from build123d import *

# Parameters (mm, degrees)
BOSS_EXTRUDE1_DEPTH     = 46
CUT_EXTRUDE1_DEPTH      = 11
SKETCH3_R               = 12.5
CUT_EXTRUDE2_DEPTH      = 300.311710429
SKETCH4_R               = 12.5
BOSS_EXTRUDE2_DEPTH     = 5
CUT_EXTRUDE3_DEPTH      = 301.796442798
CUT_EXTRUDE3_DEPTH_BACK = 301.796442798
SKETCH5_R               = 12.75


with BuildPart() as part:
    # Sketch1 → Boss-Extrude1 (new body)
    with BuildSketch(Plane(origin=(0, 0, 0), x_dir=(1, 0, 0), z_dir=(0, 1, 0))):
        with BuildLine():
            Line((0, 92.5), (190, 92.5))
            ThreePointArc((190, 92.5), (282.5, 0), (190, -92.5))
            Line((190, -92.5), (0, -92.5))
            ThreePointArc((0, -92.5), (-92.5, 0), (0, 92.5))
        make_face()
    extrude(amount=BOSS_EXTRUDE1_DEPTH)

    # Sketch2 → Cut-Extrude1 (cut)
    with BuildSketch(Plane.XZ):
        with BuildLine():
            Line((80, -92.5), (80, -22.5))
            ThreePointArc((80, -22.5), (57.5, 0), (80, 22.5))
            Line((80, 22.5), (80, 92.5))
            Line((80, 92.5), (102.5, 92.5))
            Line((102.5, 92.5), (102.5, 22.5))
            ThreePointArc((102.5, 22.5), (125, 0), (102.5, -22.5))
            Line((102.5, -22.5), (102.5, -92.5))
            Line((102.5, -92.5), (80, -92.5))
        make_face()
    extrude(amount=-CUT_EXTRUDE1_DEPTH, mode=Mode.SUBTRACT)

    # Sketch3 → Cut-Extrude2 (cut, through all)
    with BuildSketch(Plane.XZ.offset(-11)):
        with Locations(Location((91.25, 0, 0), (0, 0, 270))):
            Circle(SKETCH3_R)
    extrude(amount=-CUT_EXTRUDE2_DEPTH, mode=Mode.SUBTRACT)

    # Sketch4 → Boss-Extrude2 (add)
    with BuildSketch(Plane(origin=(0, 46, 0), x_dir=(1, 0, 0), z_dir=(0, 1, 0))):
        with BuildLine():
            ThreePointArc((102.089515, 21.8501808), (124.589515, -0.6498192), (102.089515, -23.1498192))
            Line((102.089515, -23.1498192), (79.589515, -23.1498192))
            ThreePointArc((79.589515, -23.1498192), (57.089515, -0.6498192), (79.589515, 21.8501808))
            Line((79.589515, 21.8501808), (102.089515, 21.8501808))
        make_face()
        with Locations(Location((91.25, 0, 0), (0, 0, 90))):
            Circle(SKETCH4_R, mode=Mode.SUBTRACT)
    extrude(amount=BOSS_EXTRUDE2_DEPTH)

    # Sketch5 → Cut-Extrude3 (cut, two sides: drawn at the far end of the back side and taken through both)
    with BuildSketch(Plane(origin=(0, 46, 0), x_dir=(1, 0, 0), z_dir=(0, 1, 0)).offset(-CUT_EXTRUDE3_DEPTH_BACK)):
        with Locations(Location((1.25, 0, 0), (0, 0, 270))):
            Circle(SKETCH5_R)
        with Locations(Location((181.25, 0, 0), (0, 0, 270))):
            Circle(SKETCH5_R)
    extrude(amount=CUT_EXTRUDE3_DEPTH + CUT_EXTRUDE3_DEPTH_BACK, mode=Mode.SUBTRACT)


solid = part.part
Geometry check sheet. Reference: the model listing, model coordinates, mm. A direction names the side the tool comes from. Coordinates: 2 decimals unless noted, no trailing zeros. Order: outer loops, then holes, each group sorted by start corner. A loop starts at its lowest first (then second) coordinate and runs counter-clockwise, first axis right, second up. Notation, with made-up numbers: (78, 51.5) - (114, 51.5) arc R17 cw to (114, 71.5) - close; hole circle Ø11 at (-16.75, 82). An arc over 180 degrees is marked (long way). Answer in a Markdown table with one row per item. Add a question column.
1) Cross-section at B-B, the plane x = 181.25. Record the cut outline in (y, z), then the cut area to 3 significant figures.
2) Gauge pin test, flat ends, axial feed: P1, Ø5, axis at y = 31.5, z = 70.5, coming from the +X side; P2, Ø5, axis at x = 244, y = 18.5, coming from the +Z side; P3, Ø1, axis at y = 41, z = -34, coming from the -X side. Record the tip position at first contact, or that the pin passes through.
3) Material ranges on line 1 along X through (y, z) = (42, 0); line 2 along Z through (x, y) = (91, 29); line 3 along Z through (x, y) = (1.25, 30), recorded low to high. Write a range as [from, to].
4) Release check for a two-part mould opening along X. For faces 1 (the flat face through (96, 23, 92.5)), 2 (the cylindrical face through (282.478, 22.678, -2.034)), 3 (the cylindrical face through (57.095, 48.465, 1.145)), 4 (the cylindrical face through (57.505, 5.423, -0.495)) record: +X half, -X half, draft (parallel to the pull), parting line (faces both ways), or undercut.
5) Cross-section at A-A, the plane y = 6. Record the cut outline in (x, z), then the cut area to 3 significant figures.
6) Set-up check for faces 5 (the flat face through (77, 11, 1)), 6 (the cylindrical face through (124.584, 48.465, 0.155)), 7 (the flat face through (102.5, 5, -57)): record each of +Z, -Z, +X, -X, +Y, -Y from which the full face is reachable in a straight line by a thin tool's end or side.
7) Cross-section at C-C, the plane y = 22. Record the cut outline in (x, z).
8) Cross-section at D-D, the plane z = 0. Record the cut outline in (x, y).
Check result:
| question | item | result |
|---|---|---|
| 1 | outline | (0, -92.5) - (46, -92.5) - (46, -12.75) - (0, -12.75) - close; (0, 12.75) - (46, 12.75) - (46, 92.5) - (0, 92.5) - close |
| 1 | area | 7,340 mm² |
| 2 | P1 | stops at x = 252.71 |
| 2 | P2 | stops at z = 76.84 |
| 2 | P3 | stops at x = -86.22 |
| 3 | line 1 | x = [-92.5, -11.5], [14, 78.75], [103.75, 168.5], [194, 282.5] |
| 3 | line 2 | z = [-92.5, -12.5], [12.5, 92.5] |
| 3 | line 3 | z = [-92.5, -12.75], [12.75, 92.5] |
| 4 | face 1 | draft |
| 4 | face 2 | +X half |
| 4 | face 3 | -X half |
| 4 | face 4 | undercut |
| 5 | outline | (0, -92.5) - (80, -92.5) - (80, -22.5) arc R22.5 cw to (80, 22.5) - (80, 92.5) - (0, 92.5) arc R92.5 ccw to start; (102.5, -92.5) - (190, -92.5) arc R92.5 ccw to (190, 92.5) - (102.5, 92.5) - (102.5, 22.5) arc R22.5 cw to (102.5, -22.5) - close; hole circle Ø25.5 at (1.25, 0); hole circle Ø25.5 at (181.25, 0) |
| 5 | area | 55,300 mm² |
| 6 | face 5 | -Y |
| 6 | face 6 | +X, +Y |
| 6 | face 7 | +Z, -Z, -Y |
| 7 | outline | (0, -92.5) - (190, -92.5) arc R92.5 ccw to (190, 92.5) - (0, 92.5) arc R92.5 ccw to start; hole circle Ø25.5 at (1.25, 0); hole circle Ø25 at (91.25, 0); hole circle Ø25.5 at (181.25, 0) |
| 8 | outline | (-92.5, 0) - (-11.5, 0) - (-11.5, 46) - (-92.5, 46) - close; (14, 0) - (57.5, 0) - (57.5, 11) - (78.75, 11) - (78.75, 51) - (57.1, 51) - (57.1, 46) - (14, 46) - close; (103.75, 11) - (125, 11) - (125, 0) - (168.5, 0) - (168.5, 46) - (124.58, 46) - (124.58, 51) - (103.75, 51) - close; (194, 0) - (282.5, 0) - (282.5, 46) - (194, 46) - close |
